```python
from build123d import *

# Parameters (mm, degrees)
F2_R          = 5
F3_R          = 1
F4_DEPTH      = 2.001
F4_DEPTH_BACK = 13.001


with BuildPart() as f1:
    # F0 (on Top) → F1 (revolve)
    with BuildSketch(Plane.XY):
        Polygon((-5, 0), (-3.2, 0), (-2.7, 15), (-20, 15), (-20, 13), (-5, 13), align=None)
    revolve(axis=Axis((0, -0.5978257842, 0), (0, -1, 0)))

    # F2
    f2_edges = [f1.edges().sort_by_distance(p)[0] for p in [
        (5, 13, 0),
    ]]
    fillet(f2_edges, radius=F2_R)

    # F3 (on face) → F4 (cut, two sides)
    with BuildSketch(Plane.XZ.offset(-13)) as f4_sk:
        with Locations((7, 0)):
            Circle(F3_R)
    extrude(amount=-F4_DEPTH, mode=Mode.SUBTRACT)
    extrude(f4_sk.sketch, amount=F4_DEPTH_BACK, mode=Mode.SUBTRACT)


solid = f1.part
```
Here's how the part is built. I have some questions about the finished solid (model axes, mm). A direction names the side the tool comes from. Coordinates: 2 decimals unless noted, no trailing zeros. Loops run counter-clockwise (first coordinate to the right, second up) from the corner with the lowest first, then second, coordinate; pieces in that order, holes last. Notation, with made-up numbers: M -35.75,45.5 L 1.25,45.5 A33 cw 1.25,78.5 Z; hole C 70,86 d6. An arc over 180 degrees is marked long. One line per item, written item: value.
1. Imagine slicing it at C-C (y = 2.75). List the corners of the cut face in (x, z) for me, and give its area (3 significant figures).
Geometry says:
outline: C 0,0 d10; hole C 0,0 d6.22
area: 48.2 mm2
2. Please list where these lines run through material, in increasing order: probe 1 along Y at (x, z) = (11, 3); probe 2 along X at (y, z) = (12, 0); probe 3 along X at (y, z) = (11.9, 0).
Geometry says:
probe 1: y = 13 to 15
probe 2: x = -7 to -2.8, 2.8 to 6
probe 3: x = -6.87 to -2.8, 2.8 to 6
3. Imagine slicing it at A-A (x = 0). List the corners of the cut face in (y, z) for me, and give its area (3 significant figures).
Geometry says:
outline: M 0,-5 L 8,-5 A5 cw 13,-10 L 13,-20 L 15,-20 L 15,-2.7 L 0,-3.2 Z; M 0,3.2 L 15,2.7 L 15,20 L 13,20 L 13,10 A5 cw 8,5 L 0,5 Z
area: 132 mm2
4. Imagine slicing it at B-B (z = 0). List the corners of the cut face in (x, y) for me, and give its area (3 significant figures).
Geometry says:
outline: M -20,13 L -10,13 A5 cw -5,8 L -5,0 L -3.2,0 L -2.7,15 L -20,15 Z; M 2.7,15 L 3.2,0 L 5,0 L 5,8 A5 cw 6,11 L 6,15 Z; M 8,12.58 A5 cw 10,13 L 20,13 L 20,15 L 8,15 Z
area: 126 mm2
5. Will these pins go through, and if not, where does the flat tip stop? pin 1 Ø4 at (y, z) = (9.5, 4.5) entering from -X; pin 2 Ø6 at (y, z) = (6, -1.5) entering from +X; pin 3 Ø8 at (y, z) = (4.5, -6.5) entering from -X.
Geometry says:
pin 1: stops at x = -5.11
pin 2: stops at x = 5.05
pin 3: stops at x = -4.33
6. Imagine slicing it at D-D (x = 13.5). List the corners of the cut face in (y, z) for me, and give its area (3 significant figures).
Geometry says:
outline: M 13,-14.76 L 15,-14.76 L 15,14.76 L 13,14.76 Z
area: 59.0 mm2
7. Thinking about a two-plate mould opening in Z: for faces 3 (the conical face through (0.639, 7.605, 2.876)), 4 (the cylindrical face through (4.336, 13.986, 19.524)), 5 (the flat face through (5, 13, -9)), which applies, +Z half, -Z half, draft (parallel to the pull), parting line (faces both ways), or undercut?
Geometry says:
face 3: undercut
face 4: parting line
face 5: draft
8. On a 3-axis mill with a long thin cutter (end or side, diameter ignored), from which of +Z, -Z, +X, -X, +Y, -Y can I reach the whole of each face in a straight line? I mean faces 1 (the flat face through (-3.3, 0, 1)), 2 (the cylindrical face through (1.08, 3.94, 4.88)). Say none if no direction works.
Geometry says:
face 1: +Z, -Z, +X, -X, -Y
face 2: -Y
